Verification items for the finished model (mm, model axes). Face numbers are marked on the shaded views. A direction names the side the tool comes from. Round coordinates to 2 decimals unless told otherwise and drop trailing zeros. Write each loop counter-clockwise with the first axis right and the second up, starting at its lowest first coordinate (ties: lowest second). Pieces come first, ordered by that corner, then holes. Notation, with made-up numbers: (25, 69.25) -> (57, 69.25) arc R11 cw to (57, 73.25) -> close; hole circle Ø7 at (35.5, 80). An arc over 180 degrees is marked (long way). Use CSV: the item, a comma, the result in double quotes.
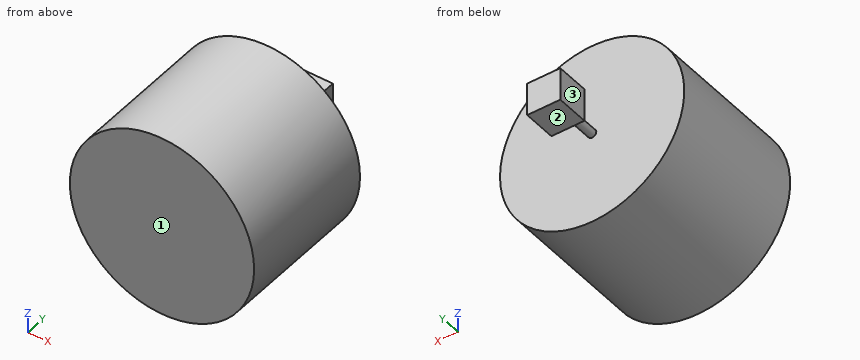
```python
from build123d import *

# Parameters (mm, degrees)
ESQUISSE1_R      = 223
EXTRUSION1_DEPTH = 350
ESQUISSE2_R      = 10
EXTRUSION2_DEPTH = 80
ESQUISSE3_W      = 80
ESQUISSE3_H      = 80
EXTRUSION3_DEPTH = 80


with BuildPart() as part:
    # Esquisse1 → Extrusion1 (new body)
    with BuildSketch(Plane(origin=(0, 0, 0), x_dir=(1, 0, 0), z_dir=(0, 1, 0))):
        Circle(ESQUISSE1_R)
    extrude(amount=EXTRUSION1_DEPTH)

    # Esquisse2 → Extrusion2 (add)
    with BuildSketch(Plane(origin=(0, 350, 0), x_dir=(1, 0, 0), z_dir=(0, 1, 0))):
        Circle(ESQUISSE2_R)
    extrude(amount=EXTRUSION2_DEPTH)

    # Esquisse3 → Extrusion3 (add)
    with BuildSketch(Plane(origin=(0, 430, 0), x_dir=(1, 0, 0), z_dir=(0, 1, 0))):
        Rectangle(ESQUISSE3_W, ESQUISSE3_H)
    extrude(amount=EXTRUSION3_DEPTH)


solid = part.part
```
Q1. Section check A-A (z = 0). Record the cut outline in (x, y), plus the area to 3 significant figures.
Filled in:
outline,"(-223, 0) -> (223, 0) -> (223, 350) -> (10, 350) -> (10, 430) -> (40, 430) -> (40, 510) -> (-40, 510) -> (-40, 430) -> (-10, 430) -> (-10, 350) -> (-223, 350) -> close"
area,"164,000 mm²"
Q2. Section check B-B (x = 24). Record the cut outline in (y, z), plus the area to 3 significant figures.
Filled in:
outline,"(0, -221.7) -> (350, -221.7) -> (350, 221.7) -> (0, 221.7) -> close; (430, -40) -> (510, -40) -> (510, 40) -> (430, 40) -> close"
area,"162,000 mm²"
Q3. Section check D-D (x = -61.5). Record the cut outline in (y, z).
Filled in:
outline,"(0, -214.35) -> (350, -214.35) -> (350, 214.35) -> (0, 214.35) -> close"
Q4. Go/stop test with flat-tipped pins: P1, Ø4, axis at x = 59.5, y = 114.5, coming from the +Z side; P2, Ø24, axis at x = -11.5, y = 455, coming from the +Z side; P3, Ø4, axis at x = -142.5, z = -116.5, coming from the +Y side. Record where each tip stops, or that it passes through.
Filled in:
P1,"z = 215.46"
P2,"z = 40"
P3,"y = 350"
Q5. Section check C-C (y = 409.5). Record the cut outline in (x, z).
Filled in:
outline,"circle Ø20 at (0, 0)"
Q6. Material ranges on L1, parallel to Y at x = 110, z = -14; L2, parallel to Z at x = -198, y = 199; L3, parallel to Z at x = -202.5, y = 73, recorded low to high.
Filled in:
L1,"0 to 350"
L2,"-102.59 to 102.59"
L3,"-93.4 to 93.4"
Q7. Access from +Z, -Z, +X, -X, +Y, -Y to the whole of each face (thin tool, end or side, straight path). Record for the marked faces 1, 2 and 3.
Filled in:
face 1,"+Z, -Z, +X, -X, -Y"
face 2,"-Z, +X, -X, +Y"
face 3,"+Z, -Z, -X, +Y"
